Read the model definition and answer for the solid it produces. Units are mm, in the model's axes. A direction names the side the tool comes from. Give positions to 0.01 mm unless a question says otherwise; leave off trailing zeros. Write each loop counter-clockwise with the first axis right and the second up, starting at its lowest first coordinate (ties: lowest second). Pieces come first, ordered by that corner, then holes. Notation, with made-up numbers: (74.25, 57.5) - (106.25, 57.5) arc R13 cw to (106.25, 64.5) - close; hole circle Ø5 at (77, 60.25). An arc over 180 degrees is marked (long way). Answer as CSV lines item,"result".
```python
from build123d import *

# Parameters (mm, degrees)
SKETCH1_R           = 16
SKETCH1_R_2         = 9
SKETCH1_R_3         = 7.5
BOSS_EXTRUDE1_DEPTH = 27.5
BOSS_EXTRUDE2_START = 2
SKETCH1_3_R         = 9
SKETCH1_3_R_2       = 7.5
BOSS_EXTRUDE2_DEPTH = 2
BOSS_EXTRUDE3_START = -27.5
SKETCH1_4_R         = 9
SKETCH1_4_R_2       = 7.5
BOSS_EXTRUDE3_DEPTH = 2
SKETCH2_R           = 1.5
CUT_EXTRUDE1_DEPTH  = 38.17862289


with BuildPart() as part:
    # Sketch1 → Boss-Extrude1 (new body)
    # profile 1 of 2: a face of its own
    with BuildSketch(Plane.XY):
        Circle(SKETCH1_R)
        Circle(SKETCH1_R_2, mode=Mode.SUBTRACT)
    # profile 2 of 2: a face of its own
    with BuildSketch(Plane.XY):
        Circle(SKETCH1_R_2)
        Circle(SKETCH1_R_3, mode=Mode.SUBTRACT)
    extrude(amount=-BOSS_EXTRUDE1_DEPTH)

    # Sketch1<3> → Boss-Extrude2 (add)
    with BuildSketch(Plane.XY.offset(BOSS_EXTRUDE2_START)):
        Circle(SKETCH1_3_R)
        Circle(SKETCH1_3_R_2, mode=Mode.SUBTRACT)
    extrude(amount=-BOSS_EXTRUDE2_DEPTH)

    # Sketch1<4> → Boss-Extrude3 (add)
    with BuildSketch(Plane.XY.offset(BOSS_EXTRUDE3_START)):
        Circle(SKETCH1_4_R)
        Circle(SKETCH1_4_R_2, mode=Mode.SUBTRACT)
    extrude(amount=-BOSS_EXTRUDE3_DEPTH)

    # Sketch2 → Cut-Extrude1 (cut, through all)
    with BuildSketch(Plane.XY):
        with Locations((-8.485281374, 8.485281374)):
            Circle(SKETCH2_R)
        with Locations((8.485281374, 8.485281374)):
            Circle(SKETCH2_R)
        with Locations((8.485281374, -8.485281374)):
            Circle(SKETCH2_R)
        with Locations((-8.485281374, -8.485281374)):
            Circle(SKETCH2_R)
    extrude(amount=-CUT_EXTRUDE1_DEPTH, mode=Mode.SUBTRACT)


solid = part.part
```
(1) For faces 1 (the cylindrical face through (-7.493, 0.33, -13.53)), 2 (the flat face through (7, -7, 0)), 3 (the cylindrical face through (-1.172, 8.923, -28.486)), determine the directions among +Z, -Z, +X, -X, +Y, -Y from which every point of the face is accessible in a straight line to the end or side of a thin tool.
Worked out:
face 1,"+Z, -Z"
face 2,"+Z"
face 3,"-Z"
(2) Each of these flat-tipped pins is pushed along its axis until it touches: P1, Ø8, axis at x = -9, z = -5, coming from the -Y side; P2, Ø2, axis at y = 6, z = -5, coming from the +X side; P3, Ø1, axis at x = 5.5, z = -19.5, coming from the +Y side; P4, Ø1, axis at y = 0.5, z = -18.5, coming from the +X side. Where does it stop, or does it pass through?
Worked out:
P1,"stops at y = -15.2"
P2,"stops at x = 15.2"
P3,"stops at y = 15.2"
P4,"stops at x = 16"
(3) A cutting plane is placed at A-A (y = 0). Write down the section's boundary in (x, z).
Worked out:
outline,"(-16, -27.5) - (-9, -27.5) - (-9, -29.5) - (-7.5, -29.5) - (-7.5, 2) - (-9, 2) - (-9, 0) - (-16, 0) - close; (7.5, -29.5) - (9, -29.5) - (9, -27.5) - (16, -27.5) - (16, 0) - (9, 0) - (9, 2) - (7.5, 2) - close"
(4) The mould has two halves that part along Y. Classify faces 4 (the cylindrical face through (-1.172, 8.923, 1.014)), 5 (the cylindrical face through (8.16, -9.95, -13.56)), 6 (the flat face through (-2, 7.4, 2)): +Y half, -Y half, draft (parallel to the pull), parting line (faces both ways), or undercut.
Worked out:
face 4,"parting line"
face 5,"undercut"
face 6,"draft"
(5) Find the intervals of material crossed by L1, parallel to Y at x = -9.5, z = -13; L2, parallel to Y at x = 9, z = -3.5, in increasing order.
Worked out:
L1,"y = -12.87 to -9.59, -7.38 to 7.38, 9.59 to 12.87"
L2,"y = -13.23 to -9.89, -7.08 to 7.08, 9.89 to 13.23"
(6) A cutting plane is placed at C-C (y = -8). Write down the section's boundary in (x, z).
Worked out:
outline,"(-13.86, -27.5) - (-9.9, -27.5) - (-9.9, 0) - (-13.86, 0) - close; (-7.07, -27.5) - (-4.12, -27.5) - (-4.12, -29.5) - (4.12, -29.5) - (4.12, -27.5) - (7.07, -27.5) - (7.07, 0) - (4.12, 0) - (4.12, 2) - (-4.12, 2) - (-4.12, 0) - (-7.07, 0) - close; (9.9, -27.5) - (13.86, -27.5) - (13.86, 0) - (9.9, 0) - close"
